from build123d import *

# Parameters (mm, degrees)
F2_R = 10


with BuildPart() as f1:
    # F0 (on Top) → F1 (revolve)
    with BuildSketch(Plane.XY):
        with BuildLine():
            Line((-5.5, 20), (-5.5, 10))
            ThreePointArc((-5.5, 10), (-11.951506, 6.74352), (-14.549876, 0))
            Line((-14.549876, 0), (-14.049876, 0))
            ThreePointArc((-14.049876, 0), (-11.427303, 6.573629), (-5, 9.536777))
            Line((-5, 9.536777), (-5, 20))
            Line((-5, 20), (-35, 90))
            Line((-35, 90), (-35.5, 90))
            Line((-35.5, 90), (-5.5, 20))
        make_face()
    revolve(axis=Axis((0, 34.304306, 0), (0, -1, 0)))

    # F2
    f2_edges = [f1.edges().sort_by_distance(p)[0] for p in [
        (5.5, 10, 0),
        (5.5, 20, 0),
        (5, 9.536777, 0),
        (5, 20, 0),
    ]]
    fillet(f2_edges, radius=F2_R)


solid = f1.part
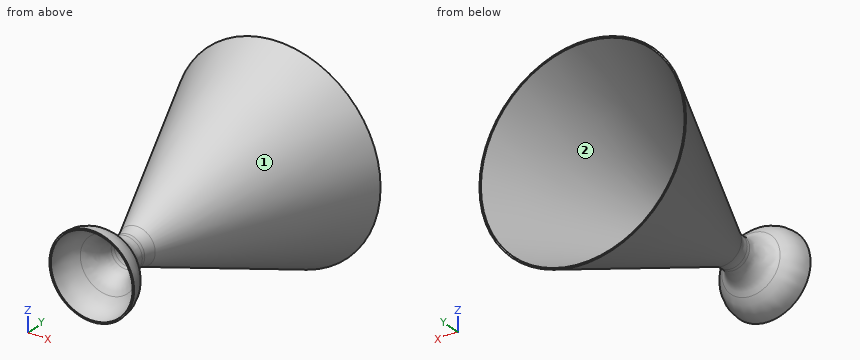
Geometry check sheet. Reference: the model listing, model coordinates, mm. Face numbers are marked on the shaded views. Round coordinates to 2 decimals unless told otherwise and drop trailing zeros. Order: outer loops, then holes, each group sorted by start corner. A loop starts at its lowest first (then second) coordinate and runs counter-clockwise, first axis right, second up. Notation, with made-up numbers: (33, 29) - (47, 29) arc R12 cw to (47, 50) - close; hole circle Ø7 at (18, 49). An arc over 180 degrees is marked (long way). One line per question, with ' | ' between items. Start each with the question number.
(1) Release check for a two-part mould opening along X. For the marked faces 1 and 2 record: released by +X, released by -X, zero draft, split by the parting line, or undercut.
(2) Sectioned sample at B-B on y = 58. Record the cut outline in (x, z), and give its area (3 significant figures).
(3) Thickness scan on L1, parallel to Z at x = 0, y = 17.1; L2, parallel to Z at x = -6, y = 10. Record the ranges inside material, lowest first. Write a range as [from, to].
(4) Sectioned sample at A-A on y = 34. Record the cut outline in (x, z), and give its area (3 significant figures).
(5) Depth check by flat-ended pin: pin 1 Ø1 at (x, z) = (25.5, 3.5) entering from +Y; pin 2 Ø6 at (x, z) = (-28, 11) entering from -Y; pin 3 Ø6 at (x, y) = (11, 65) entering from -Z. Enter the tip coordinate at first touch or a pass-through.
Conclusion:
1) face 1: split by the parting line | face 2: undercut
2) outline: circle Ø43.57 at (0, 0); hole circle Ø42.57 at (0, 0) | area: 67.7 mm2
3) L1: z = [-5.5, -5], [5, 5.5] | L2: z = [-5.49, -4.32], [4.32, 5.49]
4) outline: circle Ø23 at (0, 0); hole circle Ø22 at (0, 0) | area: 35.3 mm2
5) pin 1: stops at y = 69.56 | pin 2: stops at y = 70.36 | pin 3: stops at z = -24.12
